from build123d import *

# Parameters (mm, degrees)
F1_START      = 78.8
F0_R          = 32.5
F0_R_2        = 5
F1_DEPTH      = 1.2
F2_DEPTH      = 80
F2_DEPTH_BACK = 15
F3_DEPTH      = 1.2
F4_START      = -13.8
F4_DEPTH      = 1.2
F5_D          = 5
F5_DEPTH      = 15.001
F6_D          = 5
F6_DEPTH      = 12
F6_TIP        = 1.5021515476
F8_D          = 5
F8_DEPTH      = 32.501
F9_D          = 5


with BuildPart() as f1:
    # F0 (on Top) → F1 (new body)
    with BuildSketch(Plane.XY.offset(F1_START)):
        Circle(F0_R)
        with Locations((0, -25)):
            Circle(F0_R_2, mode=Mode.SUBTRACT)
        with Locations((0, 25)):
            Circle(F0_R_2, mode=Mode.SUBTRACT)
    extrude(amount=F1_DEPTH)

    # F0 (on Top) → F2 (join, two sides)
    with BuildSketch(Plane.XY) as f2_sk:
        with Locations((0, 25)):
            Circle(F0_R_2)
        with Locations((0, -25)):
            Circle(F0_R_2)
    extrude(amount=F2_DEPTH)
    extrude(f2_sk.sketch, amount=-F2_DEPTH_BACK)

    # F0 (on Top) → F3 (join)
    with BuildSketch(Plane.XY):
        Circle(F0_R)
        with Locations((0, -25)):
            Circle(F0_R_2, mode=Mode.SUBTRACT)
        with Locations((0, 25)):
            Circle(F0_R_2, mode=Mode.SUBTRACT)
    extrude(amount=F3_DEPTH)

    # F0 (on Top) → F4 (join)
    with BuildSketch(Plane.XY.offset(F4_START)):
        Circle(F0_R)
        with Locations((0, -25)):
            Circle(F0_R_2, mode=Mode.SUBTRACT)
        with Locations((0, 25)):
            Circle(F0_R_2, mode=Mode.SUBTRACT)
    extrude(amount=-F4_DEPTH)

    # F5 (through all, one way)
    with BuildSketch(Plane.XY):
        with Locations((0, -32.5)):
            Circle(F5_D / 2)
    extrude(amount=-F5_DEPTH, mode=Mode.SUBTRACT)

    # F6
    with Locations(Plane(origin=(0, 0, 0), x_dir=(1, 0, 0), z_dir=(0, 0, -1))):
        with Locations((0, 32.5)):
            Hole(F6_D / 2, depth=F6_DEPTH)
            with Locations((0, 0, -(F6_DEPTH + F6_TIP / 2))):  # 118° drill point
                Cone(0, F6_D / 2, F6_TIP, mode=Mode.SUBTRACT)

    # F8 (through all, one way)
    with BuildSketch(Plane.XZ):
        with Locations((0, 40)):
            Circle(F8_D / 2)
    extrude(amount=-F8_DEPTH, mode=Mode.SUBTRACT)

    # F9 (through all)
    with Locations(Plane(origin=(0, 0, 0), x_dir=(1, 0, 0), z_dir=(0, 1, 0))):
        with Locations((0, -40)):
            Hole(F9_D / 2)


solid = f1.part
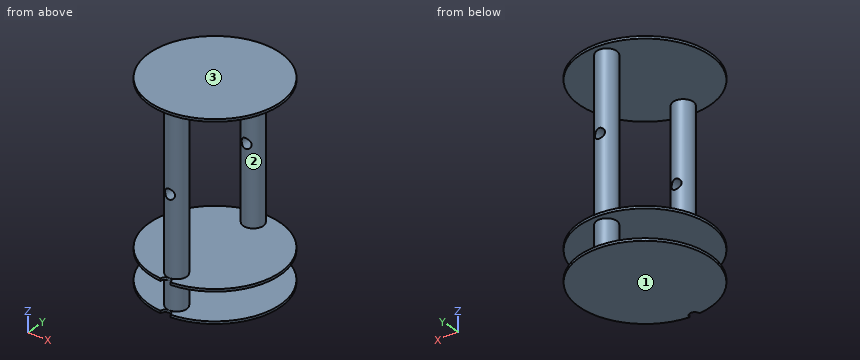
Geometry: final body of the model. Coordinates: model frame, mm. Face numbers are marked on the shaded views. Coordinates: 2 decimals unless noted, no trailing zeros. Loops run counter-clockwise (first coordinate to the right, second up) from the corner with the lowest first, then second, coordinate; pieces in that order, holes last. Notation, with made-up numbers: M -9,-23.75 L 45,-23.75 A17 ccw 45,-12.75 Z; hole C -20.5,44 d8. An arc over 180 degrees is marked long. One line per item, written item: value. Start each with the question number.
1) Cut plane A-A (y = -16.5). Return loops of the section in (x, z).
2) Cut plane C-C (z = 40). Return loops of the section in (x, y), then the cut area to 3 significant figures.
3) Cut plane B-B (x = -10.5). Return loops of the section in (y, z), then the cut area to 3 significant figures.
4) Material intervals for L1, parallel to Z at x = -27, y = -16; L2, parallel to Y at x = 0, z = 58.5; L3, parallel to Z at x = 0, y = 23.5, sorted ascending. Write a range as from..to.
5) Pin query (flat end, axial travel): P1, Ø6, axis at x = 3.5, z = 34, coming from the -Y side; P2, Ø10, axis at y = -17.5, z = 39.5, coming from the -X side; P3, Ø6, axis at x = -6, z = 45.5, coming from the -Y side. Return the tip coordinate at first contact, or that it passes through.
6) Cut plane D-D (z = 70.5). Return loops of the section in (x, y), then the cut area to 3 significant figures.
7) Draft query along Z for the marked faces 1, 2 and 3. Return one class per face: released by +Z, released by -Z, zero draft, split by the parting line, or undercut.
Evaluation:
1. outline: M -28,-15 L 28,-15 L 28,-13.8 L -28,-13.8 Z; M -28,0 L 28,0 L 28,1.2 L -28,1.2 Z; M -28,78.8 L 28,78.8 L 28,80 L -28,80 Z
2. outline: M -2.5,-29.33 L -2.5,-20.67 A5 ccw Z; M -2.5,20.67 L -2.5,29.33 A5 ccw Z; M 2.5,-29.33 A5 ccw 2.5,-20.67 Z; M 2.5,20.67 A5 ccw 2.5,29.33 Z
2. area: 61.4 mm^2
3. outline: M -30.76,-15 L 30.76,-15 L 30.76,-13.8 L -30.76,-13.8 Z; M -30.76,0 L 30.76,0 L 30.76,1.2 L -30.76,1.2 Z; M -30.76,78.8 L 30.76,78.8 L 30.76,80 L -30.76,80 Z
3. area: 221 mm^2
4. L1: -15..-13.8, 0..1.2, 78.8..80
4. L2: -30..-20, 20..30
4. L3: -15..37.5, 42.5..80
5. P1: y = -29.97
5. P2: x = -4.33
5. P3: y = -29
6. outline: C 0,-25 d10; C 0,25 d10
6. area: 157 mm^2
7. face 1: released by -Z
7. face 2: undercut
7. face 3: released by +Z
